Source: three-view drawing plus pictorial views. Frame: mm from the lowest corner of the part. Coordinates: 2 decimals unless noted, no trailing zeros. Write each loop counter-clockwise with the first axis right and the second up, starting at its lowest first coordinate (ties: lowest second). Pieces come first, ordered by that corner, then holes. Notation, with made-up numbers: (87.5, -1) -> (104.5, -1) arc R12 cw to (104.5, 12) -> close; hole circle Ø3 at (38.25, 43). An arc over 180 degrees is marked (long way). One line per item, written item: value.
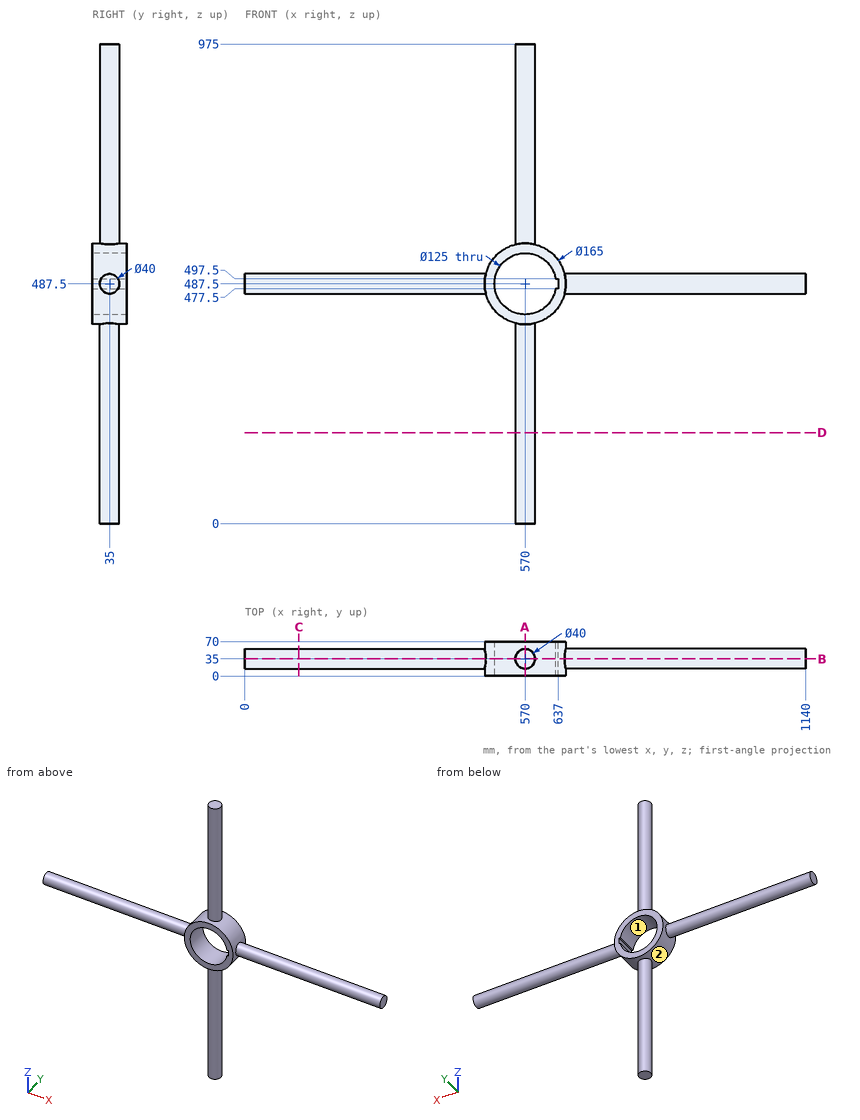
(1) Line query: line 1 (Z direction, x = 570, y = 43.5); line 2 (X direction, y = 33, z = 76); line 3 (X direction, y = 14, z = 447). Output: solid intervals per line, ascending. Write a range as [from, to].
Responses:
line 1: z = [0, 425], [550, 975]
line 2: x = [550.1, 589.9]
line 3: x = [498.13, 522.4], [617.6, 641.87]
(2) First-contact query: pin 1 (3 mm diameter, centred on y = 50, z = 350.5, fed in from +X); pin 2 (6 mm diameter, centred on x = 633.5, y = 35.5, fed in from +Z); pin 3 (4 mm diameter, centred on x = 494, y = 17.5, fed in from +Z). Flat tips, straight axial feed; report the tip coordinate or a pass-through.
Responses:
pin 1: stops at x = 584.76
pin 2: stops at z = 543.59
pin 3: stops at z = 523.97
(3) Section A-A (x = 570). Return the cut outline in (y, z), then the cut area to 3 significant figures.
Responses:
outline: (0, 405) -> (15, 405) -> (15, 0) -> (55, 0) -> (55, 405) -> (70, 405) -> (70, 425) -> (0, 425) -> close; (0, 550) -> (70, 550) -> (70, 570) -> (55, 570) -> (55, 975) -> (15, 975) -> (15, 570) -> (0, 570) -> close
area: 35,200 mm2
(4) Section B-B (y = 35). Return the cut outline in (x, z), then the cut area to 3 significant figures.
Responses:
outline: (0, 467.5) -> (489.96, 467.5) arc R82.5 ccw to (550, 407.46) -> (550, 0) -> (590, 0) -> (590, 407.46) arc R82.5 ccw to (650.04, 467.5) -> (1140, 467.5) -> (1140, 507.5) -> (650.04, 507.5) arc R82.5 ccw to (590, 567.54) -> (590, 975) -> (550, 975) -> (550, 567.54) arc R82.5 ccw to (489.96, 507.5) -> (0, 507.5) -> close; hole (631.69, 477.5) -> (637, 477.5) -> (637, 497.5) -> (631.69, 497.5) arc R62.5 ccw (long way) to start
area: 80,500 mm2
(5) Section D-D (z = 185). Return the cut outline in (x, y), then the cut area to 3 significant figures.
Responses:
outline: circle Ø40 at (570, 35)
area: 1,260 mm2
(6) Section C-C (x = 110). Return the cut outline in (y, z).
Responses:
outline: circle Ø40 at (35, 487.5)
(7) Pull-direction query (Z, two-part tool) for the marked faces 1 and 2; classes: released by +Z, released by -Z, zero draft, split by the parting line, or undercut.
Responses:
face 1: undercut
face 2: split by the parting line
